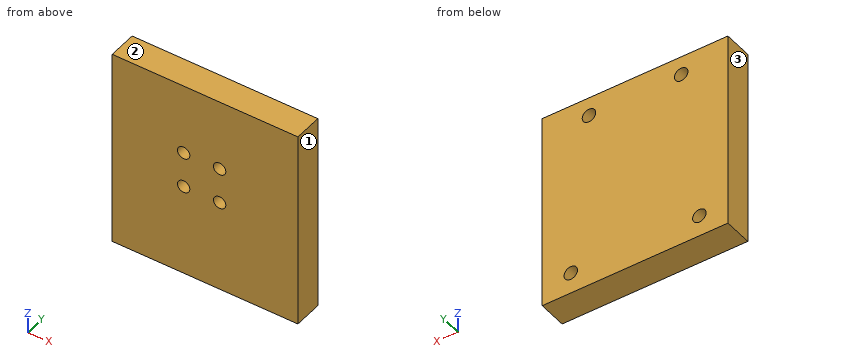
from build123d import *

# Parameters (mm, degrees)
SKETCH1_W           = 82.55
SKETCH1_H           = 88.9
BOSS_EXTRUDE1_DEPTH = 12.7
SKETCH2_R           = 3
CUT_EXTRUDE1_DEPTH  = 6.35
SKETCH3_R           = 2.75
CUT_EXTRUDE2_DEPTH  = 6.35


with BuildPart() as part:
    # Sketch1 → Boss-Extrude1 (new body)
    with BuildSketch(Plane(origin=(0, 0, 0), x_dir=(1, 0, 0), z_dir=(0, 1, 0))):
        with Locations((-41.275, -44.45)):
            Rectangle(SKETCH1_W, SKETCH1_H)
    extrude(amount=BOSS_EXTRUDE1_DEPTH)

    # Sketch2 → Cut-Extrude1 (cut)
    with BuildSketch(Plane(origin=(0, 12.7, 0), x_dir=(1, 0, 0), z_dir=(0, 1, 0))):
        with Locations(Location((-69.85, -9.525, 0), (0, 0, 270))):
            Circle(SKETCH2_R)
        with Locations(Location((-12.7, -9.525, 0), (0, 0, 270))):
            Circle(SKETCH2_R)
        with Locations(Location((-61.775, -80.504650473, 0), (0, 0, 270))):
            Circle(SKETCH2_R)
        with Locations(Location((-20.775, -80.504650473, 0), (0, 0, 270))):
            Circle(SKETCH2_R)
    extrude(amount=-CUT_EXTRUDE1_DEPTH, mode=Mode.SUBTRACT)

    # Sketch3 → Cut-Extrude2 (cut)
    with BuildSketch(Plane.XZ):
        with Locations(Location((-50.8, 57.15, 0), (0, 0, 270))):
            Circle(SKETCH3_R)
        with Locations(Location((-34.8, 57.15, 0), (0, 0, 270))):
            Circle(SKETCH3_R)
        with Locations(Location((-50.8, 41.15, 0), (0, 0, 270))):
            Circle(SKETCH3_R)
        with Locations(Location((-34.8, 41.15, 0), (0, 0, 270))):
            Circle(SKETCH3_R)
    extrude(amount=-CUT_EXTRUDE2_DEPTH, mode=Mode.SUBTRACT)


solid = part.part
Could you check a few things on this model? Use its own coordinates, in mm. Face numbers are marked on the shaded views. Give positions to 0.01 mm unless a question says otherwise; leave off trailing zeros. Order: outer loops, then holes, each group sorted by start corner. A loop starts at its lowest first (then second) coordinate and runs counter-clockwise, first axis right, second up. Notation, with made-up numbers: M -19.5,15 L 38.5,15 A24 cw 38.5,30 Z; hole C 62,-38 d2. An arc over 180 degrees is marked long. One line per question, with ' | ' between items.
1. I'm going to push flat-ended pins straight in: pin 1 (1.6 mm diameter, centred on x = -51.5, z = 41.5, fed in from -Y); pin 2 (1.8 mm diameter, centred on x = -20, z = 82, fed in from +Y). Where does each tip first touch, or does it pass through?
Results:
pin 1: y = 6.35 | pin 2: y = 6.35
2. I want a section at A-A (z = 41.15). List the corners of the cut face in (x, y) for me.
Results:
outline: M -82.55,0 L -53.55,0 L -53.55,6.35 L -48.05,6.35 L -48.05,0 L -37.55,0 L -37.55,6.35 L -32.05,6.35 L -32.05,0 L 0,0 L 0,12.7 L -82.55,12.7 Z
3. If I drill on line 1 (X direction, y = 3, z = 57.15); line 2 (Z direction, x = -70, y = 7); line 3 (Y direction, x = -50, z = 59), over which ranges is the centre line in solid material (lowest first)?
Results:
line 1: -82.55 to -53.55, -48.05 to -37.55, -32.05 to 0 | line 2: 0 to 6.53, 12.52 to 88.9 | line 3: 6.35 to 12.7
4. I want a section at C-C (y = 11). List the corners of the cut face in (x, z) for me (3 decimals).
Results:
outline: M -82.55,0 L 0,0 L 0,88.9 L -82.55,88.9 Z; hole C -69.85,9.525 d6; hole C -61.775,80.505 d6; hole C -20.775,80.505 d6; hole C -12.7,9.525 d6
5. I want a section at B-B (x = -12.7). List the corners of the cut face in (y, z) for me (3 decimals), and give its area (3 significant figures).
Results:
outline: M 0,0 L 12.7,0 L 12.7,6.525 L 6.35,6.525 L 6.35,12.525 L 12.7,12.525 L 12.7,88.9 L 0,88.9 Z | area: 1,090 mm²
6. I want a section at D-D (x = -34.8). List the corners of the cut face in (y, z) for me, and give its area (3 significant figures).
Results:
outline: M 0,0 L 12.7,0 L 12.7,88.9 L 0,88.9 L 0,59.9 L 6.35,59.9 L 6.35,54.4 L 0,54.4 L 0,43.9 L 6.35,43.9 L 6.35,38.4 L 0,38.4 Z | area: 1,060 mm²
7. We'd pull the mould along X, two halves only. Please class the marked faces 1, 2 and 3: +X half, -X half, draft (parallel to the pull), parting line (faces both ways), or undercut.
Results:
face 1: +X half | face 2: draft | face 3: -X half
